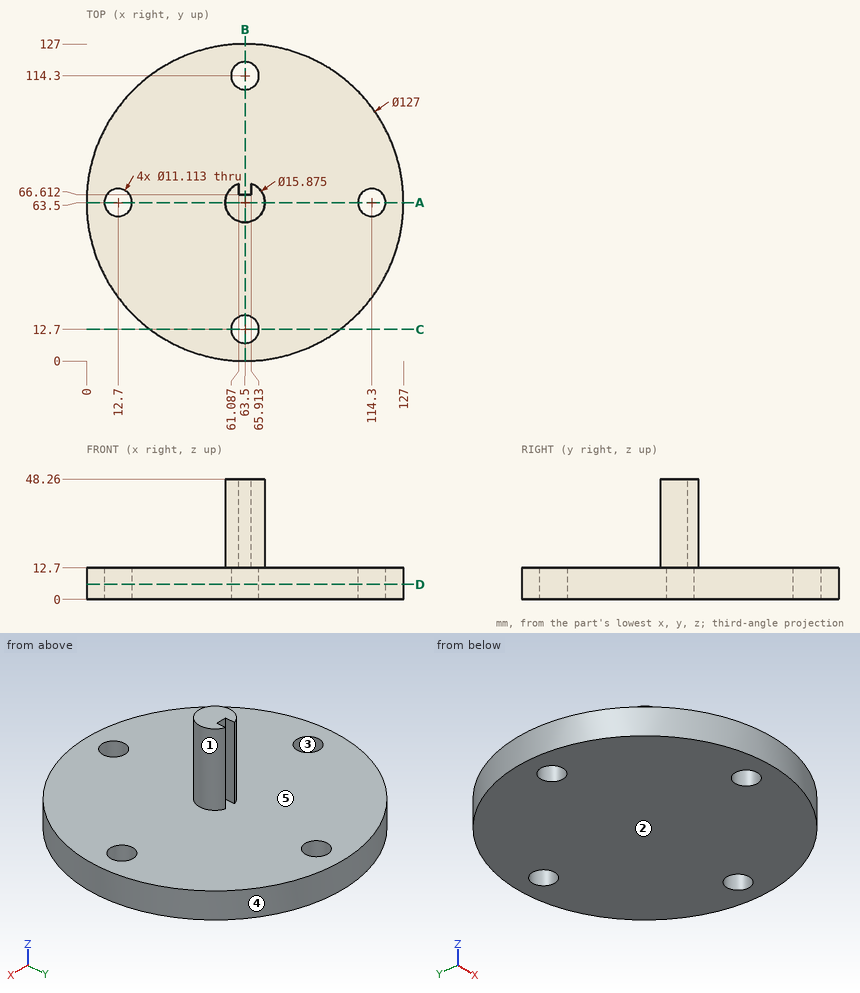
Check sheet for the drawn part. Datum: minimum x, y, z corner. Units: mm. A direction names the side the tool comes from. Round coordinates to 2 decimals unless told otherwise and drop trailing zeros. Order: outer loops, then holes, each group sorted by start corner. A loop starts at its lowest first (then second) coordinate and runs counter-clockwise, first axis right, second up.
1) Tool access check on the marked faces 1 and 2. Record the directions out of +Z, -Z, +X, -X, +Y, -Y that give a thin tool (end or side, any length) a straight path to the whole face; none if there is none.
2) Section check B-B (x = 63.5). Record the boundary of the cut face in (y, z).
3) Go/stop test with flat-tipped pins: pin 1 Ø10 at (x, y) = (54.5, 113.5) entering from +Z; pin 2 Ø3 at (x, y) = (34, 45) entering from -Z; pin 3 Ø2 at (x, z) = (79.5, 8) entering from -Y; pin 4 Ø2.5 at (x, z) = (64, 23) entering from +Y. Record where each tip stops, or that it passes through.
4) Section check C-C (y = 12.7). Record the boundary of the cut face in (x, z).
5) Mould release check, pull along Y, two halves, no side actions. Record for the marked faces 3, 4 and 5: +Y half, -Y half, draft (parallel to the pull), parting line (faces both ways), or undercut.
6) Section check A-A (y = 63.5). Record the boundary of the cut face in (x, z).
7) Section check D-D (z = 6). Record the boundary of the cut face in (x, y), and give its area (3 significant figures).
8) Scan lines: line 1 (X direction, y = 63, z = 7); line 2 (Y direction, x = 63.5, z = 3.75); line 3 (Z direction, x = 93.5, y = 112.5). Record each from-to range of solid material in increasing order.
Result:
1. face 1: +Z
1. face 2: -Z, +X, -X, +Y, -Y
2. outline: (0, 0) - (7.14, 0) - (7.14, 12.7) - (0, 12.7) - close; (18.26, 0) - (108.74, 0) - (108.74, 12.7) - (66.61, 12.7) - (66.61, 48.26) - (55.56, 48.26) - (55.56, 12.7) - (18.26, 12.7) - close; (119.86, 0) - (127, 0) - (127, 12.7) - (119.86, 12.7) - close
3. pin 1: stops at z = 12.7
3. pin 2: stops at z = 0
3. pin 3: stops at y = 1.8
3. pin 4: stops at y = 66.61
4. outline: (25.4, 0) - (57.94, 0) - (57.94, 12.7) - (25.4, 12.7) - close; (69.06, 0) - (101.6, 0) - (101.6, 12.7) - (69.06, 12.7) - close
5. face 3: undercut
5. face 4: parting line
5. face 5: draft
6. outline: (0, 0) - (7.14, 0) - (7.14, 12.7) - (0, 12.7) - close; (18.26, 0) - (108.74, 0) - (108.74, 12.7) - (71.44, 12.7) - (71.44, 48.26) - (55.56, 48.26) - (55.56, 12.7) - (18.26, 12.7) - close; (119.86, 0) - (127, 0) - (127, 12.7) - (119.86, 12.7) - close
7. outline: circle Ø127 at (63.5, 63.5); hole circle Ø11.11 at (12.7, 63.5); hole circle Ø11.11 at (63.5, 12.7); hole circle Ø11.11 at (63.5, 114.3); hole circle Ø11.11 at (114.3, 63.5)
7. area: 12,300 mm2
8. line 1: x = 0 to 7.17, 18.23 to 108.77, 119.83 to 127
8. line 2: y = 0 to 7.14, 18.26 to 108.74, 119.86 to 127
8. line 3: z = 0 to 12.7
